Answer from the drawing. Dimensions are ordinates in mm from the lowest x, y and z of the part. A direction names the side the tool comes from. Give positions to 0.01 mm unless a question says otherwise; leave off trailing zeros. Write each loop counter-clockwise with the first axis right and the second up, starting at its lowest first coordinate (ties: lowest second). Pieces come first, ordered by that corner, then holes.
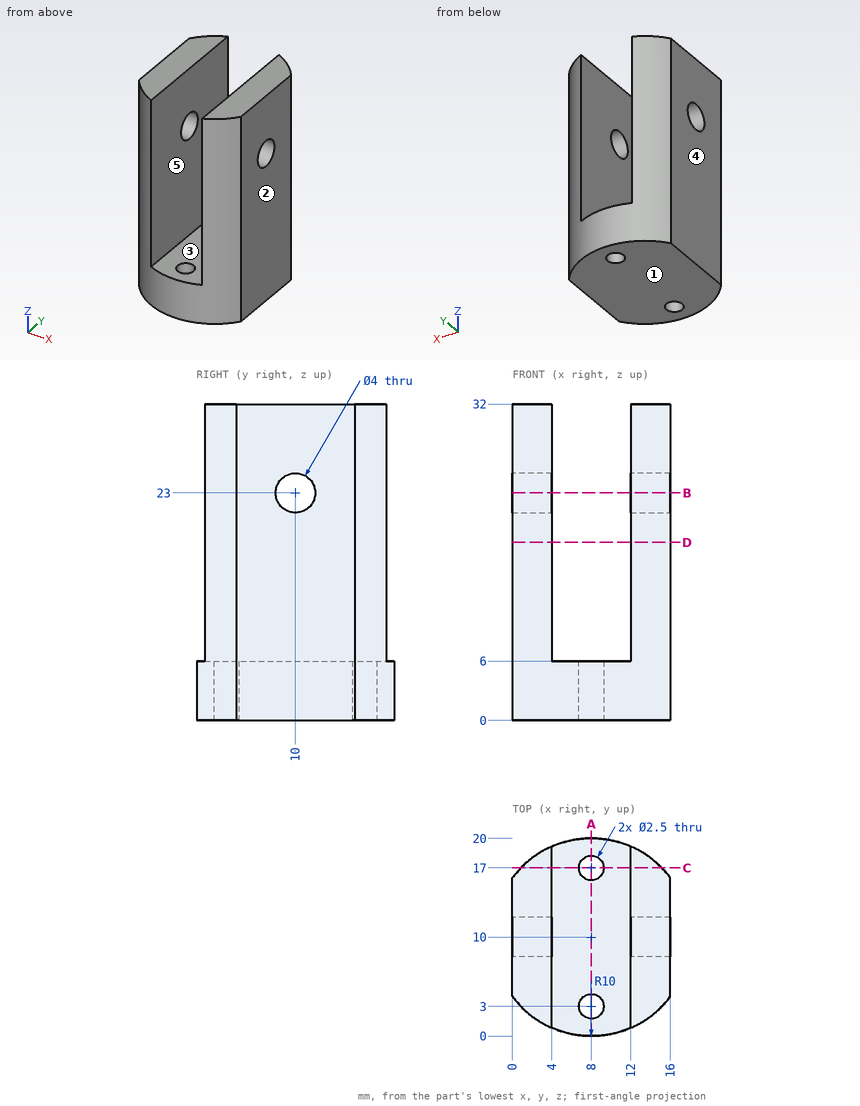
Item 1: Which of the six approach directions +Z, -Z, +X, -X, +Y, -Y give full straight-line access (tool end or side, diameter ignored) to the marked faces 4 and 5?
Result set:
face 4: +Z, -Z, -X, +Y, -Y
face 5: +Z, +Y, -Y
Item 2: Find the intervals of material crossed by line 1 along Z through (x, y) = (14.8, 10); line 2 along X through (y, z) = (4.25, 27); line 3 along Z through (x, y) = (11.75, 18.25), in increasing order.
Result set:
line 1: z = 0 to 21, 25 to 32
line 2: x = 0 to 4, 12 to 16
line 3: z = 0 to 6
Item 3: Section D-D (z = 18) is taken. Write down the section's boundary in (x, y).
Result set:
outline: (0, 4) arc R10 ccw to (4, 0.83) - (4, 19.17) arc R10 ccw to (0, 16) - close; (12, 0.83) arc R10 ccw to (16, 4) - (16, 16) arc R10 ccw to (12, 19.17) - close
Item 4: Each of these flat-tipped pins is pushed along its axis until it touches: pin 1 Ø3 at (y, z) = (18, 7.5) entering from -X; pin 2 Ø3 at (x, y) = (8, 17) entering from +Z; pin 3 Ø1 at (x, z) = (4, 18) entering from +Y. Where does it stop, or does it pass through?
Result set:
pin 1: stops at x = 0.4
pin 2: stops at z = 6
pin 3: stops at y = 19.17
Item 5: Section C-C (y = 17) is taken. Write down the section's boundary in (x, z).
Result set:
outline: (0.86, 0) - (6.75, 0) - (6.75, 6) - (4, 6) - (4, 32) - (0.86, 32) - close; (9.25, 0) - (15.14, 0) - (15.14, 32) - (12, 32) - (12, 6) - (9.25, 6) - close
Item 6: Section B-B (z = 23) is taken. Write down the section's boundary in (x, y), and give its area (3 significant figures).
Result set:
outline: (0, 4) arc R10 ccw to (4, 0.83) - (4, 8) - (0, 8) - close; (0, 12) - (4, 12) - (4, 19.17) arc R10 ccw to (0, 16) - close; (12, 0.83) arc R10 ccw to (16, 4) - (16, 8) - (12, 8) - close; (12, 12) - (16, 12) - (16, 16) arc R10 ccw to (12, 19.17) - close
area: 93.8 mm2
Item 7: Determine the mould class of the marked faces 1, 2 and 3 for opening direction X: pulls with the +X half, pulls with the -X half, needs draft (parallel to the pull), parting line crosses it, or undercut.
Result set:
face 1: needs draft
face 2: pulls with the +X half
face 3: undercut
Item 8: Section A-A (x = 8) is taken. Write down the section's boundary in (y, z), and give its area (3 significant figures).
Result set:
outline: (0, 0) - (1.75, 0) - (1.75, 6) - (0, 6) - close; (4.25, 0) - (15.75, 0) - (15.75, 6) - (4.25, 6) - close; (18.25, 0) - (20, 0) - (20, 6) - (18.25, 6) - close
area: 90.0 mm2
